```python
from build123d import *

# Parameters (mm, degrees)
SKETCH1_W            = 3
SKETCH1_H            = 16
BOSS_EXTRUDE1_DEPTH  = 25
BOSS_EXTRUDE2_DEPTH  = 25
M2_CLEARANCE_HOLE1_D = 2.4
CHAMFER1_SIZE        = 4
SKETCH12_W           = 4
SKETCH12_H           = 3.5
SKETCH12_R           = 1.2
CUT_EXTRUDE1_DEPTH   = 5


with BuildPart() as part:
    # Sketch1 → Boss-Extrude1 (new body)
    with BuildSketch(Plane.XY):
        Rectangle(SKETCH1_W, SKETCH1_H)
    extrude(amount=BOSS_EXTRUDE1_DEPTH)

    # Sketch4 → Boss-Extrude2 (add, through all)
    with BuildSketch(Plane.XY.offset(25)):
        Polygon((1.5, 8), (9.5, 0), (1.5, -8), align=None)
    extrude(amount=-BOSS_EXTRUDE2_DEPTH)

    # M2 Clearance Hole1 (through all)
    with Locations(Plane(origin=(-1.5, 0, 0), x_dir=(0, 0, -1), z_dir=(-1, 0, 0))):
        with Locations((-2, -6.25), (-23, 6.25), (-23, -6.25), (-2, 6.25)):
            Hole(M2_CLEARANCE_HOLE1_D / 2)

    # Chamfer1
    chamfer1_edges = [part.edges().sort_by_distance(p)[0] for p in [
        (9.5, 0, 12.5),
    ]]
    chamfer(chamfer1_edges, length=CHAMFER1_SIZE)

    # Sketch8 → Ø6.0mm Dowel Hole3 (revolve, cut)
    with BuildSketch(Plane(origin=(2.671572875, 0, 25), x_dir=(0, -1, 0), z_dir=(1, 0, 0))):
        Polygon((0, 0), (0, 9.802581857), (3, 8), (3, 0), align=None)
    f_6_0mm_dowel_hole3 = revolve(axis=Axis((2.671572875, 0, 31.35), (0, 0, -1)), mode=Mode.SUBTRACT)

    # Mirror2: Ø6.0mm Dowel Hole3 across plane
    add(f_6_0mm_dowel_hole3.mirror(Plane.XY.offset(12.5)), mode=Mode.SUBTRACT)

    # Sketch12 → Cut-Extrude1 (cut)
    with BuildSketch(Plane(origin=(6.671572875, 0, 0), x_dir=(0, 0, -1), z_dir=(1, 0, 0))):
        with Locations((-2, 6.25)):
            Rectangle(SKETCH12_W, SKETCH12_H)
        with Locations((-2, 6.25)):
            Circle(SKETCH12_R, mode=Mode.SUBTRACT)
        with Locations((-2, 6.25)):
            Circle(SKETCH12_R)
        with Locations((-2, -6.25)):
            Circle(SKETCH12_R)
        with Locations((-2, -6.25)):
            Rectangle(SKETCH12_W, SKETCH12_H)
        with Locations((-2, -6.25)):
            Circle(SKETCH12_R, mode=Mode.SUBTRACT)
        with Locations((-23, -6.25)):
            Circle(SKETCH12_R)
        with Locations((-23, -6.25)):
            Rectangle(SKETCH12_W, SKETCH12_H)
        with Locations((-23, -6.25)):
            Circle(SKETCH12_R, mode=Mode.SUBTRACT)
        with Locations((-23, 6.25)):
            Circle(SKETCH12_R)
        with Locations((-23, 6.25)):
            Rectangle(SKETCH12_W, SKETCH12_H)
        with Locations((-23, 6.25)):
            Circle(SKETCH12_R, mode=Mode.SUBTRACT)
    extrude(amount=-CUT_EXTRUDE1_DEPTH, mode=Mode.SUBTRACT)


solid = part.part
```
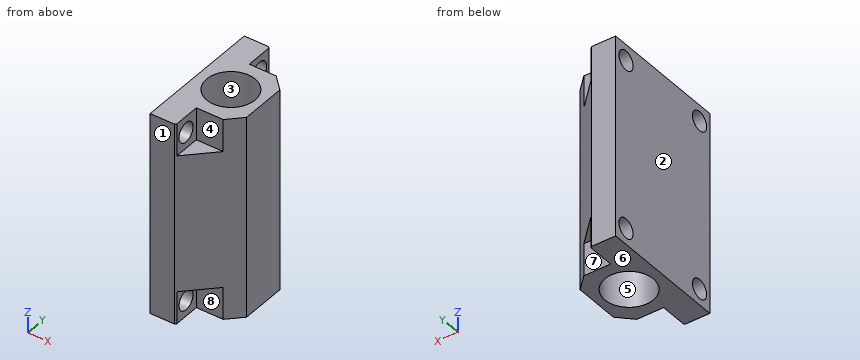
Source: CAD feature listing. Evaluate the final solid. Frame: model axes, mm. Face numbers are marked on the shaded views. A direction names the side the tool comes from. Coordinates: 2 decimals unless noted, no trailing zeros. Order: outer loops, then holes, each group sorted by start corner. A loop starts at its lowest first (then second) coordinate and runs counter-clockwise, first axis right, second up. Notation, with made-up numbers: (49, 5.25) - (108, 5.25) arc R17 ccw to (108, 34.25) - close; hole circle Ø8 at (41.25, 51). An arc over 180 degrees is marked (long way). One line per item, written item: value.
1) Reachability of the marked faces 4, 5, 6, 7 and 8 from +Z, -Z, +X, -X, +Y, -Y: full face, straight path, thin tool, end or side. Return the list, or none.
Computed values:
face 4: +Z, +X, -Y
face 5: -Z
face 6: -Z, +X, -X, +Y, -Y
face 7: -Z, +X, +Y
face 8: -Z, +X, -Y
2) Cut plane A-A on y = 6.25. Output: boundary loops of the cut face in (x, z), plus the area to 3 significant figures.
Computed values:
outline: (-1.5, 0) - (1.67, 0) - (1.67, 0.8) - (-1.5, 0.8) - close; (-1.5, 3.2) - (1.67, 3.2) - (1.67, 4) - (3.25, 4) - (3.25, 21) - (1.67, 21) - (1.67, 21.8) - (-1.5, 21.8) - close; (-1.5, 24.2) - (1.67, 24.2) - (1.67, 25) - (-1.5, 25) - close
area: 90.9 mm^2
3) Cut plane B-B on z = 23. Output: boundary loops of the cut face in (x, y), plus the area to 3 significant figures.
Computed values:
outline: (-1.5, -8) - (1.5, -8) - (1.67, -7.83) - (1.67, -7.45) - (-1.5, -7.45) - close; (-1.5, -5.05) - (1.67, -5.05) - (1.67, -4.5) - (5, -4.5) - (6.67, -2.83) - (6.67, 2.83) - (5, 4.5) - (1.67, 4.5) - (1.67, 5.05) - (-1.5, 5.05) - close; (-1.5, 7.45) - (1.67, 7.45) - (1.67, 7.83) - (1.5, 8) - (-1.5, 8) - close; hole circle Ø6 at (2.67, 0)
area: 49.4 mm^2
4) Contact query for flat-ended pins moving along their axis: pin 1 (3.5 mm diameter, centred on x = 2.67, y = 0, fed in from +Z); pin 2 (1.7 mm diameter, centred on x = 4, z = 2, fed in from +Y); pin 3 (2 mm diameter, centred on y = -6.25, z = 23, fed in from +X); pin 4 (1.7 mm diameter, centred on y = -7, z = 22.5, fed in from +X). Output: stop coordinate, or through.
Computed values:
pin 1: stops at z = 16.25
pin 2: stops at y = 4.5
pin 3: passes through
pin 4: stops at x = 1.67
5) Ray query, line 1 (Z direction, x = 0.25, y = -6.25); line 2 (Z direction, x = 1.5, y = 5.25); line 3 (Y direction, x = 0.7, z = 2). Return the intervals inside material, ascending. Write a range as [from, to].
Computed values:
line 1: z = [0, 0.8], [3.2, 21.8], [24.2, 25]
line 2: z = [0, 1.34], [2.66, 22.34], [23.66, 25]
line 3: y = [-8, -7.45], [-5.05, -2.26], [2.26, 5.05], [7.45, 8]
6) Cut plane C-C on z = 18.75. Output: boundary loops of the cut face in (x, y).
Computed values:
outline: (-1.5, -8) - (1.5, -8) - (6.67, -2.83) - (6.67, 2.83) - (1.5, 8) - (-1.5, 8) - close; hole circle Ø6 at (2.67, 0)
7) Mould query, pull axis X, two halves, no side actions, for the marked faces 1, 2 and 3. Classes: released by +X, released by -X, zero draft, split by the parting line, or undercut.
Computed values:
face 1: zero draft
face 2: released by -X
face 3: undercut
8) Cut plane D-D on y = -4.75. Output: boundary loops of the cut face in (x, z), plus the area to 3 significant figures.
Computed values:
outline: (-1.5, 0) - (1.67, 0) - (1.67, 4) - (4.75, 4) - (4.75, 21) - (1.67, 21) - (1.67, 25) - (-1.5, 25) - close
area: 132 mm^2
